Model file for the job. Use its own axes, mm. Coordinates: 2 decimals unless noted, no trailing zeros. Write each loop counter-clockwise with the first axis right and the second up, starting at its lowest first coordinate (ties: lowest second). Pieces come first, ordered by that corner, then holes. Notation, with made-up numbers: M 82.25,34 L 92.25,34 A20 cw 92.25,48 Z; hole C 59.5,-30 d5. An arc over 180 degrees is marked long. Put each result on its own line as item: value. Start each with the question number.
Q1. Cut at C-C (x = -22.5). Write the cut outline in (y, z), then the cut area to 3 significant figures.
Q2. Pull direction Z, two halves, no side cores. Call faces 1 (the flat face through (-1, -1, 0)), 2 (the cylindrical face through (-25.869, -18.805, 32.688)), 3 (the flat face through (-1, -33.402, 5)), 4 (the flat face through (0, 14.177, 33)): pulls with the +Z half, pulls with the -Z half, needs draft (parallel to the pull), parting line crosses it, or undercut.
Q3. Cut at A-A (x = 23). Write the cut outline in (y, z).
Q4. Drop a flat-ended pin along its axis: pin 1 (5 mm diameter, centred on x = -5, z = 29, fed in from -Y). Give the stop position or say it passes through.
Q5. Cut at D-D (z = 23). Write the cut outline in (x, y), then the cut area to 3 significant figures.
Q6. Cut at B-B (y = 11). Write the cut outline in (x, z).
Q7. Drill centre lines: line 1 along Z through (x, y) = (-1.5, -26.5); line 2 along Y through (x, z) = (0, 46.5); line 3 along Y through (x, z) = (-20.5, 17). Where is each one in solid material? Low to high.
```python
from build123d import *

# Parameters (mm, degrees)
F0_W     = 62.7262871712
F0_H     = 64.8624785244
F1_DEPTH = 67.31
F2_W     = 47.5787650794
F2_H     = 46.6077653691
F3_DEPTH = 72.644
F4_R     = 6.5399432167
F5_DEPTH = 52.07


with BuildPart() as f1:
    # F0 (on Top) → F1 (new body)
    with BuildSketch(Plane.XY):
        with Locations((-0.2912962809, -0.9709950536)):
            Rectangle(F0_W, F0_H)
    extrude(amount=F1_DEPTH)

    # F2 (on face) → F3 (cut)
    with BuildSketch(Plane.YZ.offset(31.0718473047)):
        with Locations((-9.6128517762, 33.0138341524)):
            Rectangle(F2_W, F2_H)
    extrude(amount=-F3_DEPTH, mode=Mode.SUBTRACT)

    # F4 (on face) → F5 (join)
    with BuildSketch(Plane.XY.offset(9.7099514678)):
        with Locations((-21.0486296564, -23.2247561216)):
            Circle(F4_R)
    extrude(amount=F5_DEPTH)


solid = f1.part
```
Computed values:
1. outline: M -33.4,0 L 31.46,0 L 31.46,67.31 L -33.4,67.31 L -33.4,56.32 L -29.6,56.32 L -29.6,9.71 L -33.4,9.71 Z; hole M -16.85,9.71 L 14.18,9.71 L 14.18,56.32 L -16.85,56.32 Z
1. area: 2,740 mm2
2. face 1: pulls with the -Z half
2. face 2: undercut
2. face 3: needs draft
2. face 4: undercut
3. outline: M -33.4,0 L 31.46,0 L 31.46,67.31 L -33.4,67.31 L -33.4,56.32 L 14.18,56.32 L 14.18,9.71 L -33.4,9.71 Z
4. pin 1: y = 14.18
5. outline: M -31.65,14.18 L 31.07,14.18 L 31.07,31.46 L -31.65,31.46 Z; C -21.05,-23.22 d13.08
5. area: 1,220 mm2
6. outline: M -31.65,0 L 31.07,0 L 31.07,9.71 L -31.65,9.71 Z; M -31.65,56.32 L 31.07,56.32 L 31.07,67.31 L -31.65,67.31 Z
7. line 1: 0 to 9.71, 56.32 to 67.31
7. line 2: 14.18 to 31.46
7. line 3: -29.74 to -16.71, 14.18 to 31.46
